Could you check a few things on this model? Use its own coordinates, in mm. A direction names the side the tool comes from. Coordinates: 2 decimals unless noted, no trailing zeros. Loops run counter-clockwise (first coordinate to the right, second up) from the corner with the lowest first, then second, coordinate; pieces in that order, holes last.
from build123d import *

# Parameters (mm, degrees)
SKETCH014_R     = 20
PAD010_DEPTH    = 3
SKETCH015_R     = 6
PAD011_DEPTH    = 1
SKETCH016_R     = 1.5
POCKET003_DEPTH = 5
POCKET004_DEPTH = 5


with BuildPart() as part:
    # Sketch014 → Pad010 (new body)
    with BuildSketch(Plane.XZ):
        Circle(SKETCH014_R)
    extrude(amount=PAD010_DEPTH)

    # Sketch015 (on Face2 of Pad010) → Pad011 (join)
    with BuildSketch(Plane(origin=(0, 0, 0), x_dir=(1, 0, 0), z_dir=(0, 1, 0))):
        Circle(SKETCH015_R)
    extrude(amount=PAD011_DEPTH)

    # Sketch016 (on Face5 of Pad011) → Pocket003 (cut)
    with BuildSketch(Plane(origin=(0, 1, 0), x_dir=(1, 0, 0), z_dir=(0, 1, 0))):
        Circle(SKETCH016_R)
    extrude(amount=-POCKET003_DEPTH, mode=Mode.SUBTRACT)

    # Sketch020 (on Face3 of Pocket003) → Pocket004 (cut)
    with BuildSketch(Plane.XZ.offset(3)):
        Polygon((17.052171, -11.966453), (10.195413, -11.966453), (-6.895316, -21.074684), (18.587267, -21.074684), align=None)
    extrude(amount=-POCKET004_DEPTH, mode=Mode.SUBTRACT)


with BuildPart() as part_1:
    # Body002 placement: moved
    add(part.part.moved(Location((61.4, -13.9, 30.2))))


solid = part_1.part
(1) I need wall thicknesses on probe 1 along X at (y, z) = (-15.3, 30.2); probe 2 along Y at (x, z) = (55, 16); probe 3 along Z at (x, y) = (61.4, -15.9). Which ranges of each line are inside material? Lowest first, please.
Answers:
probe 1: x = 41.4 to 59.9, 62.9 to 81.4
probe 2: y = -16.9 to -13.9
probe 3: z = 12.8 to 28.7, 31.7 to 50.2
(2) We'd pull the mould along X, two halves only. Please class faces 3 (the face through (60.29, -14.87, 29.19)), 4 (the face through (56.64, -13.41, 33.85)), 5 (the face through (57, -13.9, 35)): +X half, -X half, draft (parallel to the pull), parting line (faces both ways), or undercut.
Answers:
face 3: undercut
face 4: parting line
face 5: draft
(3) For pin 1 (1 mm diameter, centred on x = 75.5, y = -15, fed in from +Z); pin 2 (2 mm diameter, centred on x = 73.5, y = -15.5, fed in from +Z); pin 3 (3 mm diameter, centred on x = 76.5, z = 37, fed in from +Y), each with a flat end and sliding along its axis, tell me the tip position at first contact or that it passes through.
Answers:
pin 1: stops at z = 44.86
pin 2: stops at z = 46.84
pin 3: stops at y = -13.9
(4) Imagine slicing it at A-A, the plane z = 30.2. Write out the boundary of the cut face in (x, y).
Answers:
outline: (41.4, -16.9) - (59.9, -16.9) - (59.9, -12.9) - (55.4, -12.9) - (55.4, -13.9) - (41.4, -13.9) - close; (62.9, -16.9) - (81.4, -16.9) - (81.4, -13.9) - (67.4, -13.9) - (67.4, -12.9) - (62.9, -12.9) - close
(5) Imagine slicing it at C-C, the plane y = -15.75. Write out the boundary of the cut face in (x, z).
Answers:
outline: (57.31, 10.62) - (71.6, 18.23) - (77.43, 18.23) arc R20 ccw (long way) to start; hole circle Ø3 at (61.4, 30.2)
(6) Which directions (+Z, -Z, +X, -X, +Y, -Y) give clear straight access to the entire face, cutting with the end or side of a thin tool? Please do faces 1 (the face through (75, -15, 18.234)), 2 (the face through (57, -16.9, 31)).
Answers:
face 1: -Z, +X, +Y, -Y
face 2: +Z, -Z, +X, -X, -Y
(7) Imagine slicing it at B-B, the plane x = 61.4. Write out the boundary of the cut face in (y, z), and give its area (3 significant figures).
Answers:
outline: (-16.9, 12.8) - (-13.9, 12.8) - (-13.9, 24.2) - (-12.9, 24.2) - (-12.9, 28.7) - (-16.9, 28.7) - close; (-16.9, 31.7) - (-12.9, 31.7) - (-12.9, 36.2) - (-13.9, 36.2) - (-13.9, 50.2) - (-16.9, 50.2) - close
area: 112 mm2
(8) Imagine slicing it at D-D, the plane z = 35. Write out the boundary of the cut face in (x, y).
Answers:
outline: (41.98, -16.9) - (80.82, -16.9) - (80.82, -13.9) - (65, -13.9) - (65, -12.9) - (57.8, -12.9) - (57.8, -13.9) - (41.98, -13.9) - close
